Geometry: final body of the model. Coordinates: model frame, mm. Face numbers are marked on the shaded views. A direction names the side the tool comes from. Give positions to 0.01 mm unless a question says otherwise; leave off trailing zeros. Loops run counter-clockwise (first coordinate to the right, second up) from the corner with the lowest first, then second, coordinate; pieces in that order, holes last. Notation, with made-up numbers: (26, 9.5) -> (46, 9.5) arc R29 cw to (46, 40.5) -> close; hole circle Ø11 at (-36, 76). An arc over 180 degrees is marked (long way). One line per question, with ' | ' between items. Start each with the question number.
Item 1: Material intervals for line 1 along X through (y, z) = (-2, -6.75); line 2 along Z through (x, y) = (-0.65, -4.5); line 3 along Y through (x, z) = (-0.6, 3.5), sorted ascending. Write a range as [from, to].
Item 2: Section A-A on x = 0.9. Return loops of the section in (y, z), then the cut area to 3 significant figures.
Item 3: Mould query, pull axis X, two halves, no side actions, for the marked faces 1, 2 and 3. Classes: released by +X, released by -X, zero draft, split by the parting line, or undercut.
Item 4: Set-up query: the marked faces 4, 5 and 6. Return all of +Z, -Z, +X, -X, +Y, -Y with unobstructed straight access to the full face (end or side cutting, diameter ignored); none if empty.
Item 5: Pin query (flat end, axial travel): P1, Ø1, axis at y = -4.5, z = 2.5, coming from the -X side; P2, Ø1, axis at x = 1, z = -6, coming from the -Y side; P3, Ø2, axis at x = 2, y = 2.5, coming from the +Z side. Return the tip coordinate at first contact, or that it passes through.
from build123d import *

# Parameters (mm, degrees)
CHAMFER1_SIZE  = 1.27
CHAMFER1_SIZE2 = 1.513527063
FILLET1_R      = 0.254
CHAMFER3_SIZE  = 1.27
FILLET2_R      = 0.254


# Some blends are built 0.0001 mm under size
with BuildPart() as part:
    # Sketch1 → Revolve1 (revolve)
    with BuildSketch(Plane.XY, mode=Mode.PRIVATE) as revolve1_sk:
        with BuildLine():
            Line((-0.508, 7.6835), (-0.508, 6.4135))
            Line((-0.508, 6.4135), (1.524, 6.4135))
            ThreePointArc((1.524, 6.4135), (2.032, 6.6675), (2.54, 6.4135))
            Line((2.54, 6.4135), (2.54, 0))
            Line((2.54, 0), (1.27, 0))
            Line((1.27, 0), (1.27, 5.1435))
            Line((1.27, 5.1435), (-1.27, 5.1435))
            Line((-1.27, 5.1435), (-1.27, 7.6835))
            Line((-1.27, 7.6835), (-0.508, 7.6835))
        make_face()
    revolve(revolve1_sk.sketch.rotate(Axis((-6.503305215, 0, 0), (1, 0, 0)), 180), axis=Axis((-6.503305215, 0, 0), (1, 0, 0)))

    # Chamfer1
    chamfer1_edges = [part.edges().sort_by_distance(p)[0] for p in [
        (1.27, 5.1435, 0),
    ]]
    chamfer1_side = [part.faces().sort_by_distance(p)[0] for p in [
        (0, 5.1435, 0),
    ]]
    chamfer(chamfer1_edges, length=CHAMFER1_SIZE, length2=CHAMFER1_SIZE2, reference=chamfer1_side[0])

    # Fillet1
    fillet1_edges = [part.edges().sort_by_distance(p)[0] for p in [
        (2.54, 6.4135, 0),
    ]]
    fillet(fillet1_edges, radius=FILLET1_R)

    # Chamfer3
    chamfer3_edges = [part.edges().sort_by_distance(p)[0] for p in [
        (-1.27, 5.1435, 0),
    ]]
    chamfer(chamfer3_edges, length=CHAMFER3_SIZE - 0.0001)  # a hair under: the kernel refuses the full size

    # Fillet2
    # the kernel refuses this fillet: 0.254 mm, written as the material it adds along each edge
    with BuildSketch(Plane(origin=(0, 0, 0), x_dir=(0, -1, 0), z_dir=(0, 0, 1))) as fillet2_piece_1:
        with BuildLine():
            CenterArc((4.975502814, -0.190607075), FILLET2_R, 48.592790784, 1.407209216)
            Line((5.138770867, 0.003968214), (5.1435, 0))
            Line((5.1435, 0), (5.1435, -0.0001))
        make_face()
    revolve(axis=Axis((0, 0, 0), (1, 0, 0)))


solid = part.part
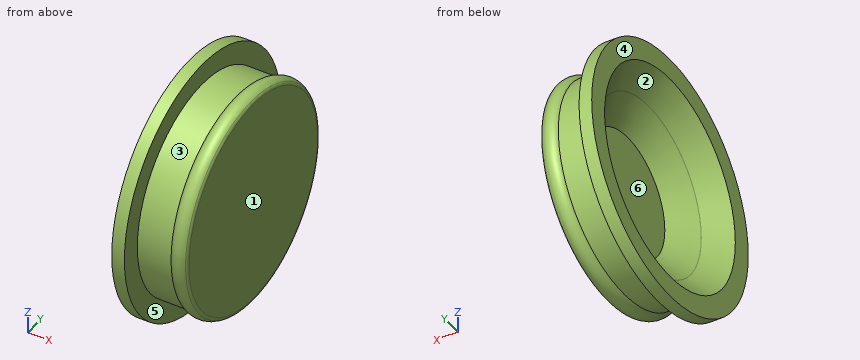
Result sheet:
1) line 1: x = [-1.27, -0.51] | line 2: z = [-6.23, -3.65], [3.65, 6.23] | line 3: y = [-6.84, -4.55], [4.55, 6.84]
2) outline: circle Ø12.83 at (0, 0); hole circle Ø8.14 at (0, 0) | area: 77.2 mm²
3) face 1: released by +X | face 2: released by -X | face 3: undercut
4) face 4: +Z, -Z, -X, +Y, -Y | face 5: none | face 6: -X
5) P1: stops at x = -0.5 | P2: stops at y = -3.3 | P3: stops at z = 6.5
